from build123d import *
from build123d import SkipClean  # not in build123d's __all__

# Parameters (mm, degrees)
F0_W     = 8.45
F0_H     = 3
F0_R     = 1.75
F0_R_2   = 1
F1_DEPTH = 1
F2_DEPTH = 2.1
F3_DEPTH = 1.8
F5_START = 1.7
F5_DEPTH = 0.3


with BuildPart() as f1:
    # F0 (on Top) → F1 (new body)
    with BuildSketch(Plane.XY):
        with Locations((29.575, -1.5)):
            Rectangle(F0_W, F0_H)
        Polygon((33.8, 0), (33.8, -3), (57.8720779386, -3), (54.8720779386, 0), align=None)
        Polygon((54.8720779386, 0), (57.8720779386, -3), (67.6, -3), (67.6, 0), align=None)
        with BuildLine():
            Line((66.8420563389, -21.7584487245), (57.7005050634, -30.9))
            Line((57.7005050634, -30.9), (67.6, -30.9))
            Line((67.6, -30.9), (67.6, -21.9))
            ThreePointArc((67.6, -21.9), (67.2144758902, -21.8643088821), (66.8420563389, -21.7584487245))
        make_face()
        with Locations((64.6, -27.9)):
            Circle(F0_R, mode=Mode.SUBTRACT)
        with BuildLine():
            Line((33.8, -3), (33.8, -30.9))
            Line((33.8, -30.9), (57.7005050634, -30.9))
            Line((57.7005050634, -30.9), (66.8420563389, -21.7584487245))
            ThreePointArc((66.8420563389, -21.7584487245), (65.5356911179, -19.4144758902), (67.6, -17.7))
            Line((67.6, -17.7), (67.6, -12.7279220614))
            Line((67.6, -12.7279220614), (57.8720779386, -3))
            Line((57.8720779386, -3), (33.8, -3))
        make_face()
        with BuildLine():
            Line((24.1, -3), (5.4852813742, -3))
            Line((5.4852813742, -3), (2.9068134786, -5.5784678956))
            ThreePointArc((2.9068134786, -5.5784678956), (2.9764254909, -5.7841452787), (3, -6))
            ThreePointArc((3, -6), (2.5378047488, -6.8430694231), (1.5784678956, -6.9068134786))
            Line((1.5784678956, -6.9068134786), (0, -8.4852813742))
            Line((0, -8.4852813742), (0, -17.7))
            ThreePointArc((0, -17.7), (2.0643088821, -19.4144758902), (0.7579436611, -21.7584487245))
            Line((0.7579436611, -21.7584487245), (9.8994949366, -30.9))
            Line((9.8994949366, -30.9), (33.8, -30.9))
            Line((33.8, -30.9), (33.8, -3))
            Line((33.8, -3), (25.35, -3))
            Line((25.35, -3), (25.35, -3.575))
            ThreePointArc((25.35, -3.575), (24.725, -4.2), (24.1, -3.575))
            Line((24.1, -3.575), (24.1, -3))
        make_face()
        with BuildLine():
            Line((9.8994949366, -30.9), (0.7579436611, -21.7584487245))
            ThreePointArc((0.7579436611, -21.7584487245), (0.3855241098, -21.8643088821), (0, -21.9))
            Line((0, -21.9), (0, -30.9))
            Line((0, -30.9), (9.8994949366, -30.9))
        make_face()
        with Locations((3, -27.9)):
            Circle(F0_R, mode=Mode.SUBTRACT)
        Polygon((8.4852813742, 0), (0, 0), (0, -3), (5.4852813742, -3), align=None)
        Polygon((24.1, 0), (8.4852813742, 0), (5.4852813742, -3), (24.1, -3), align=None)
        with BuildLine():
            Line((5.4852813742, -3), (0, -3))
            Line((0, -3), (0, -8.4852813742))
            Line((0, -8.4852813742), (1.5784678956, -6.9068134786))
            ThreePointArc((1.5784678956, -6.9068134786), (1.2928932188, -5.2928932188), (2.9068134786, -5.5784678956))
            Line((2.9068134786, -5.5784678956), (5.4852813742, -3))
        make_face()
        Polygon((67.6, -3), (57.8720779386, -3), (67.6, -12.7279220614), align=None)
        with Locations((65.6, -6)):
            Circle(F0_R_2, mode=Mode.SUBTRACT)
    extrude(amount=-F1_DEPTH)

    # F0 (on Top) → F2 (join)
    with BuildSketch(Plane.XY):
        with BuildLine():
            Line((24.1, -3), (5.4852813742, -3))
            Line((5.4852813742, -3), (2.9068134786, -5.5784678956))
            ThreePointArc((2.9068134786, -5.5784678956), (2.9764254909, -5.7841452787), (3, -6))
            ThreePointArc((3, -6), (2.5378047488, -6.8430694231), (1.5784678956, -6.9068134786))
            Line((1.5784678956, -6.9068134786), (0, -8.4852813742))
            Line((0, -8.4852813742), (0, -17.7))
            ThreePointArc((0, -17.7), (2.0643088821, -19.4144758902), (0.7579436611, -21.7584487245))
            Line((0.7579436611, -21.7584487245), (9.8994949366, -30.9))
            Line((9.8994949366, -30.9), (33.8, -30.9))
            Line((33.8, -30.9), (33.8, -3))
            Line((33.8, -3), (25.35, -3))
            Line((25.35, -3), (25.35, -3.575))
            ThreePointArc((25.35, -3.575), (24.725, -4.2), (24.1, -3.575))
            Line((24.1, -3.575), (24.1, -3))
        make_face()
    with SkipClean():  # cleaning this boolean's faces spoils the solid; the shape is the same uncleaned
        extrude(amount=-F2_DEPTH)

    # F0 (on Top) → F3 (join)
    with BuildSketch(Plane.XY):
        with BuildLine():
            Line((24.1, -3), (5.4852813742, -3))
            Line((5.4852813742, -3), (2.9068134786, -5.5784678956))
            ThreePointArc((2.9068134786, -5.5784678956), (2.9764254909, -5.7841452787), (3, -6))
            ThreePointArc((3, -6), (2.5378047488, -6.8430694231), (1.5784678956, -6.9068134786))
            Line((1.5784678956, -6.9068134786), (0, -8.4852813742))
            Line((0, -8.4852813742), (0, -17.7))
            ThreePointArc((0, -17.7), (2.0643088821, -19.4144758902), (0.7579436611, -21.7584487245))
            Line((0.7579436611, -21.7584487245), (9.8994949366, -30.9))
            Line((9.8994949366, -30.9), (33.8, -30.9))
            Line((33.8, -30.9), (33.8, -3))
            Line((33.8, -3), (25.35, -3))
            Line((25.35, -3), (25.35, -3.575))
            ThreePointArc((25.35, -3.575), (24.725, -4.2), (24.1, -3.575))
            Line((24.1, -3.575), (24.1, -3))
        make_face()
        with BuildLine():
            Line((33.8, -3), (33.8, -30.9))
            Line((33.8, -30.9), (57.7005050634, -30.9))
            Line((57.7005050634, -30.9), (66.8420563389, -21.7584487245))
            ThreePointArc((66.8420563389, -21.7584487245), (65.5356911179, -19.4144758902), (67.6, -17.7))
            Line((67.6, -17.7), (67.6, -12.7279220614))
            Line((67.6, -12.7279220614), (57.8720779386, -3))
            Line((57.8720779386, -3), (33.8, -3))
        make_face()
    extrude(amount=F3_DEPTH)

    # F4 (on Top) → F5 (cut)
    with BuildSketch(Plane.XY.offset(F5_START)):
        Polygon((8.4177003427, -20.4326654506), (12.8503657933, -15.014965108), (7.4326654506, -10.5822996573), (3, -16), align=None)
        Polygon((37.7007315866, -14.0299302159), (26.8653309013, -5.1645993147), (18, -16), (28.8354006853, -24.8653309013), align=None)
        Polygon((52.2874863017, -23.5988550582), (59.8863413599, -14.3113687565), (50.5988550582, -6.7125136983), (43, -16), align=None)
    extrude(amount=F5_DEPTH, mode=Mode.SUBTRACT)


solid = f1.part
For this review, take the finished solid that the model builds, in its own axes (mm). A direction names the side the tool comes from. Round coordinates to 2 decimals unless told otherwise and drop trailing zeros. Write each loop counter-clockwise with the first axis right and the second up, starting at its lowest first coordinate (ties: lowest second). Pieces come first, ordered by that corner, then holes. Notation, with made-up numbers: (57.25, 71) -> (111.25, 71) arc R25 ccw to (111.25, 91) -> close; hole circle Ø7 at (-8, 2.5). An arc over 180 degrees is marked (long way). Put each result on its own line as item: value.
Q1. Clearance check with flat-ended pins moving along their axes: pin 1 Ø1.4 at (x, z) = (40, 1) entering from +Y; pin 2 Ø1.2 at (y, z) = (-16.5, -2) entering from +X; pin 3 Ø3 at (x, y) = (64.6, -27.9) entering from +Z. State where each tip first meets the part, or that it passes through.
Determined:
pin 1: stops at y = -3
pin 2: stops at x = 33.8
pin 3: passes through
Q2. Consider section C-C on x = 59. State the section outline as (y, z) points.
Determined:
outline: (-30.9, -1) -> (0, -1) -> (0, 0) -> (-4.13, 0) -> (-4.13, 1.8) -> (-13.59, 1.8) -> (-13.59, 1.7) -> (-15.39, 1.7) -> (-15.39, 1.8) -> (-29.6, 1.8) -> (-29.6, 0) -> (-30.9, 0) -> close
Q3. Consider section D-D on y = -19.8. State the section outline as (x, z) points.
Determined:
outline: (2.1, -2.1) -> (33.8, -2.1) -> (33.8, -1) -> (65.5, -1) -> (65.5, 1.8) -> (55.4, 1.8) -> (55.4, 1.7) -> (47.64, 1.7) -> (47.64, 1.8) -> (32.98, 1.8) -> (32.98, 1.7) -> (22.64, 1.7) -> (22.64, 1.8) -> (8.94, 1.8) -> (8.94, 1.7) -> (7.64, 1.7) -> (7.64, 1.8) -> (2.1, 1.8) -> close
Q4. To check wall thickness, follow L1, parallel to Z at x = 58, y = -19; L2, parallel to Z at x = 26.5, y = -7; L3, parallel to Y at x = 64.5, z = -0.85. State the ranges of each line that lie inside material, in increasing order. Write a range as [from, to].
Determined:
L1: z = [-1, 1.8]
L2: z = [-2.1, 1.7]
L3: y = [-30.9, -29.65], [-26.15, 0]
Q5. The part is to be moulded in two halves that separate along Y. For faces 4 (the flat face through (51, -15, 1.7)), 5 (the flat face through (5.3, -26.3, -1.5)), 6 (the flat face through (62.8, -7.93, 0.89)), say which applies: released by +Y, released by -Y, zero draft, split by the parting line, or undercut.
Determined:
face 4: undercut
face 5: released by -Y
face 6: released by +Y
Q6. Machinability: for faces 1 (the flat face through (0.8, -7.685, -1.542)), 2 (the flat face through (28, -15, 1.7)), 3 (the flat face through (62.2, -26.4, 0.9)), which of the approach directions +Z, -Z, +X, -X, +Y, -Y give a long, thin tool a straight path to every point of the face, cutting with its end or side? Answer none if there is none.
Determined:
face 1: -Z, -X, +Y
face 2: +Z
face 3: +Z, +X, -Y
Q7. Consider section A-A on y = -27. State the section outline as (x, z) points.
Determined:
outline: (0, -1) -> (1.5, -1) -> (1.5, 0) -> (0, 0) -> close; (4.5, -1) -> (6, -1) -> (6, -2.1) -> (33.8, -2.1) -> (33.8, -1) -> (63.1, -1) -> (63.1, 0) -> (61.6, 0) -> (61.6, 1.8) -> (6, 1.8) -> (6, 0) -> (4.5, 0) -> close; (66.1, -1) -> (67.6, -1) -> (67.6, 0) -> (66.1, 0) -> close
